from build123d import *

# Parameters (mm, degrees)
MODEL_R             = 37
MODEL_R_2           = 3
BOSS_EXTRUDE1_DEPTH = 3


with BuildPart() as part:
    # Model → Boss-Extrude1 (new body)
    with BuildSketch(Plane.XY):
        Circle(MODEL_R)
        with Locations((-15, 12.5)):
            Circle(MODEL_R_2, mode=Mode.SUBTRACT)
        with Locations((-15, -12.5)):
            Circle(MODEL_R_2, mode=Mode.SUBTRACT)
        with Locations((15, -12.5)):
            Circle(MODEL_R_2, mode=Mode.SUBTRACT)
        with Locations((15, 12.5)):
            Circle(MODEL_R_2, mode=Mode.SUBTRACT)
    extrude(amount=BOSS_EXTRUDE1_DEPTH)


solid = part.part
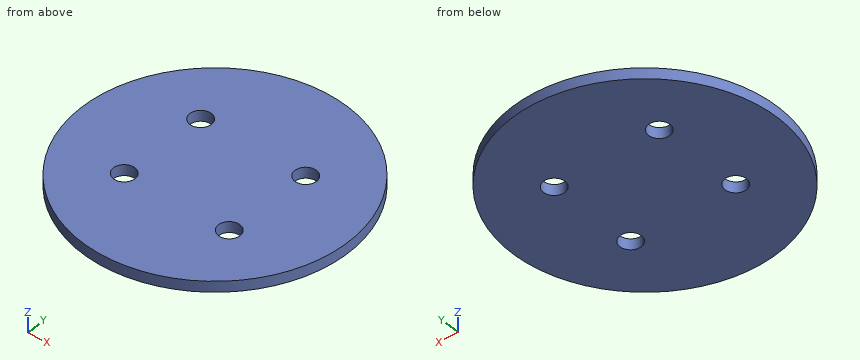
Geometry check sheet. Reference: the model listing, model coordinates, mm. Round coordinates to 2 decimals unless told otherwise and drop trailing zeros. Loops run counter-clockwise (first coordinate to the right, second up) from the corner with the lowest first, then second, coordinate; pieces in that order, holes last. Notation, with made-up numbers: (-34.5, 40) -> (-29.5, 40) arc R14 cw to (-29.5, 55) -> close; hole circle Ø10 at (58.5, -30). An arc over 180 degrees is marked (long way). Answer as a JSON object with one key per item and string values. Group by question number.
Item 1: Cross-section at C-C, the plane z = 1.85. Record the cut outline in (x, y), plus the area to 3 significant figures.
Item 2: Cross-section at A-A, the plane y = 12.5. Record the cut outline in (x, z).
Item 3: Thickness scan on line 1 along Y through (x, z) = (15, 1.85); line 2 along Y through (x, z) = (12.5, 2.8); line 3 along X through (y, z) = (13.5, 2.3). Record the ranges inside material, lowest first.
Item 4: Cross-section at D-D, the plane y = -28. Record the cut outline in (x, z), plus the area to 3 significant figures.
Item 5: Depth check by flat-ended pin: pin 1 Ø1.5 at (x, z) = (-7, 2.5) entering from +Y; pin 2 Ø1 at (x, z) = (13, 0.5) entering from -Y; pin 3 Ø5 at (x, y) = (15, 12.5) entering from +Z. Enter the tip coordinate at first touch or a pass-through.
Item 6: Cross-section at B-B, the plane x = -15. Record the cut outline in (y, z), plus the area to 3 significant figures.
Determined:
{
 "1": {"outline": "circle Ø74 at (0, 0); hole circle Ø6 at (-15, -12.5); hole circle Ø6 at (-15, 12.5); hole circle Ø6 at (15, -12.5); hole circle Ø6 at (15, 12.5)", "area": "4,190 mm²"},
 "2": {"outline": "(-34.82, 0) -> (-18, 0) -> (-18, 3) -> (-34.82, 3) -> close; (-12, 0) -> (12, 0) -> (12, 3) -> (-12, 3) -> close; (18, 0) -> (34.82, 0) -> (34.82, 3) -> (18, 3) -> close"},
 "3": {"line 1": "y = -33.82 to -15.5, -9.5 to 9.5, 15.5 to 33.82", "line 2": "y = -34.82 to -14.16, -10.84 to 10.84, 14.16 to 34.82", "line 3": "x = -34.45 to -17.83, -12.17 to 12.17, 17.83 to 34.45"},
 "4": {"outline": "(-24.19, 0) -> (24.19, 0) -> (24.19, 3) -> (-24.19, 3) -> close", "area": "145 mm²"},
 "5": {"pin 1": "stops at y = 36.47", "pin 2": "stops at y = -34.82", "pin 3": "passes through"},
 "6": {"outline": "(-33.82, 0) -> (-15.5, 0) -> (-15.5, 3) -> (-33.82, 3) -> close; (-9.5, 0) -> (9.5, 0) -> (9.5, 3) -> (-9.5, 3) -> close; (15.5, 0) -> (33.82, 0) -> (33.82, 3) -> (15.5, 3) -> close", "area": "167 mm²"}
}
